```python
from build123d import *

# Parameters (mm, degrees)
SKETCH_R     = 5
PAD_DEPTH    = 5
PAD001_DEPTH = 2.5
FILLET_R     = 5
CHAMFER_SIZE = 1.5


with BuildPart() as part:
    # Sketch → Pad (new body)
    with BuildSketch(Plane.XY):
        with BuildLine():
            Line((-50, 20), (-50, -20))
            ThreePointArc((-50, -20), (-48.535534, -23.535534), (-45, -25))
            Line((-45, -25), (45, -25))
            ThreePointArc((45, -25), (48.535534, -23.535534), (50, -20))
            Line((50, -20), (50, 20))
            ThreePointArc((50, 20), (48.535534, 23.535534), (45, 25))
            Line((45, 25), (-45, 25))
            ThreePointArc((-45, 25), (-48.535534, 23.535534), (-50, 20))
        make_face()
        with Locations((-40, 15)):
            Circle(SKETCH_R, mode=Mode.SUBTRACT)
        with Locations((40, 15)):
            Circle(SKETCH_R, mode=Mode.SUBTRACT)
        with Locations((40, -15)):
            Circle(SKETCH_R, mode=Mode.SUBTRACT)
        with Locations((-40, -15)):
            Circle(SKETCH_R, mode=Mode.SUBTRACT)
    extrude(amount=PAD_DEPTH)

    # Sketch001 → Pad001 (join, symmetric)
    with BuildSketch(Plane.XZ):
        with BuildLine():
            Line((-50, 10), (-50, 5))
            Line((-50, 5), (50, 5))
            Line((50, 5), (50, 10))
            ThreePointArc((50, 10), (44.142136, 24.142136), (30, 30))
            Line((30, 30), (-30, 30))
            ThreePointArc((-30, 30), (-44.142136, 24.142136), (-50, 10))
        make_face()
    extrude(amount=PAD001_DEPTH, both=True)

    # Fillet
    fillet_edges = [part.edges().sort_by_distance(p)[0] for p in [
        (0, -2.5, 5),
        (0, 2.5, 5),
    ]]
    fillet(fillet_edges, radius=FILLET_R)

    # Chamfer
    chamfer_edges = [part.edges().sort_by_distance(p)[0] for p in [
        (35, 15, 5),
        (-45, 15, 5),
        (35, -15, 5),
        (-45, -15, 5),
    ]]
    chamfer(chamfer_edges, length=CHAMFER_SIZE)


solid = part.part
```
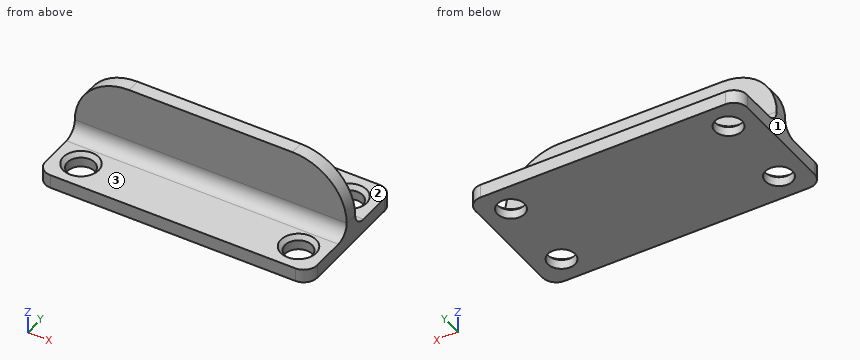
Here's how the part is built. I have some questions about the finished solid (model axes, mm). Face numbers are marked on the shaded views. A direction names the side the tool comes from. Give positions to 0.01 mm unless a question says otherwise; leave off trailing zeros. Write each loop counter-clockwise with the first axis right and the second up, starting at its lowest first coordinate (ties: lowest second). Pieces come first, ordered by that corner, then holes. Notation, with made-up numbers: (-5, -36.5) -> (5, -36.5) arc R14 cw to (5, -25.5) -> close; hole circle Ø8 at (31.5, 84). An arc over 180 degrees is marked (long way). Use one line per item in the form item = value.
1) Suppose I cut it at D-D (z = 23.5). Please give me the cut outline in (x, y).
Verdict:
outline = (-44.76, -2.5) -> (44.76, -2.5) -> (44.76, 2.5) -> (-44.76, 2.5) -> close
2) Suppose I cut it at C-C (x = 40). Please give me the cut outline in (y, z).
Verdict:
outline = (-25, 0) -> (-20, 0) -> (-20, 3.5) -> (-21.5, 5) -> (-25, 5) -> close; (-10, 0) -> (10, 0) -> (10, 3.5) -> (8.5, 5) -> (7.5, 5) arc R5 cw to (2.5, 10) -> (2.5, 27.32) -> (-2.5, 27.32) -> (-2.5, 10) arc R5 cw to (-7.5, 5) -> (-8.5, 5) -> (-10, 3.5) -> close; (20, 0) -> (25, 0) -> (25, 5) -> (21.5, 5) -> (20, 3.5) -> close
3) On a 3-axis mill with a long thin cutter (end or side, diameter ignored), from which of +Z, -Z, +X, -X, +Y, -Y can I reach the whole of each face in a straight line? I mean the marked faces 1, 2 and 3. Say none if no direction works.
Verdict:
face_1 = +Z, -Z, -X, +Y, -Y
face_2 = +Z, +X, -X, +Y
face_3 = +Z, +X, -X, -Y
4) Suppose I cut it at A-A (y = -15). Please give me the cut outline in (x, z).
Verdict:
outline = (-50, 0) -> (-45, 0) -> (-45, 3.5) -> (-46.5, 5) -> (-50, 5) -> close; (-35, 0) -> (35, 0) -> (35, 3.5) -> (33.5, 5) -> (-33.5, 5) -> (-35, 3.5) -> close; (45, 0) -> (50, 0) -> (50, 5) -> (46.5, 5) -> (45, 3.5) -> close
5) I'm going to push flat-ended pins straight in: pin 1 (8 mm diameter, centred on x = 9, z = 17.5, fed in from -Y); pin 2 (2 mm diameter, centred on x = 2, z = 12.5, fed in from +Y); pin 3 (14 mm diameter, centred on x = -12, y = 14.5, fed in from +Z). Where does each tip first touch, or does it pass through?
Verdict:
pin_1 = -2.5
pin_2 = 2.5
pin_3 = 5
6) Suppose I cut it at B-B (x = -5). Please give me the cut outline in (y, z), and give its area (3 significant figures).
Verdict:
outline = (-25, 0) -> (25, 0) -> (25, 5) -> (7.5, 5) arc R5 cw to (2.5, 10) -> (2.5, 30) -> (-2.5, 30) -> (-2.5, 10) arc R5 cw to (-7.5, 5) -> (-25, 5) -> close
area = 386 mm2
7) If I drill on L1, parallel to Y at x = -40, z = 1.3; L2, parallel to Z at x = -8.5, y = 11; L3, parallel to Y at x = 21.5, z = 25, over which ranges is the centre line in solid material (lowest first)? Write a range as [from, to].
Verdict:
L1 = [-25, -20], [-10, 10], [20, 25]
L2 = [0, 5]
L3 = [-2.5, 2.5]
